Build history of the part. All positions in model axes, mm. Face numbers are marked on the shaded views. A direction names the side the tool comes from. Round coordinates to 2 decimals unless told otherwise and drop trailing zeros. Write each loop counter-clockwise with the first axis right and the second up, starting at its lowest first coordinate (ties: lowest second). Pieces come first, ordered by that corner, then holes.
Item 1: 3-axis set-ups, long thin cutter, end or side, ignore diameter. For the marked faces 4 and 5: which of +Z, -Z, +X, -X, +Y, -Y reach the whole face in a straight line?
Item 2: Drop flat-ended pins along their axis: pin 1 Ø6 at (y, z) = (23.5, 4.5) entering from -X; pin 2 Ø0.8 at (x, z) = (0.5, 10.5) entering from -Y; pin 3 Ø0.8 at (x, y) = (-25.5, -0.5) entering from -Z. Give the stop position or say it passes through.
Item 3: Band-saw the part on C-C, the plane z = 10. Write the cut outline in (x, y), then the cut area to 3 significant figures.
Item 4: Band-saw the part on D-D, the plane x = -23. Write the cut outline in (y, z).
Item 5: Band-saw the part on A-A, the plane x = -18. Write the cut outline in (y, z), then the cut area to 3 significant figures.
Item 6: Band-saw the part on B-B, the plane y = 15. Write the cut outline in (x, z), then the cut area to 3 significant figures.
Item 7: Wall check: probe 1 along X at (y, z) = (2.4, 10); probe 2 along Z at (x, y) = (-28.5, 5.5); probe 3 along Y at (x, z) = (-2.3, 10). Give the ranges that are in metal, low to high.
Item 8: Mould opens along X. For the marked faces 1, 2 and 3 say: +X half, -X half, draft (parallel to the pull), parting line (faces both ways), or undercut.
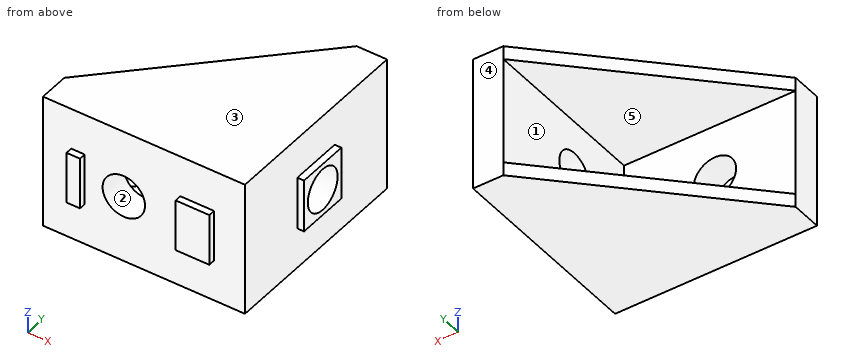
```python
from build123d import *

# Parameters (mm, degrees)
BOSS_EXTRUDE1_DEPTH = 20
CUT_EXTRUDE1_START  = -2
CUT_EXTRUDE1_DEPTH  = 16
SKETCH3_W           = 7.88
SKETCH3_H           = 7.88
BOSS_EXTRUDE2_DEPTH = 1
SKETCH4_R           = 3.15
CUT_EXTRUDE2_DEPTH  = 48.549973712
SKETCH5_W           = 2
SKETCH5_H           = 7.7
SKETCH5_W_2         = 5
BOSS_EXTRUDE3_DEPTH = 1
SKETCH6_R           = 3.15
CUT_EXTRUDE3_DEPTH  = 47.904157598


with BuildPart() as part:
    # Sketch1 → Boss-Extrude1 (new body)
    with BuildSketch(Plane.XY):
        Polygon((0, 0), (0, 30), (-4.5, 30), (-30, 4.5), (-30, 0), align=None)
    extrude(amount=BOSS_EXTRUDE1_DEPTH)

    # Sketch2 → Cut-Extrude1 (cut)
    with BuildSketch(Plane.XY.offset(20).offset(CUT_EXTRUDE1_START)):
        Polygon((-30, 4.5), (-4.5, 4.5), (-4.5, 30), align=None)
    extrude(amount=-CUT_EXTRUDE1_DEPTH, mode=Mode.SUBTRACT)

    # Sketch3 → Boss-Extrude2 (add)
    with BuildSketch(Plane(origin=(0, 0, 0), x_dir=(0, 0, -1), z_dir=(1, 0, 0))):
        with Locations((-10, 15)):
            Rectangle(SKETCH3_W, SKETCH3_H)
    extrude(amount=BOSS_EXTRUDE2_DEPTH)

    # Sketch4 → Cut-Extrude2 (cut, through all)
    with BuildSketch(Plane(origin=(1, 0, 0), x_dir=(0, 0, -1), z_dir=(1, 0, 0))):
        with Locations((-10, 15)):
            Circle(SKETCH4_R)
    extrude(amount=-CUT_EXTRUDE2_DEPTH, mode=Mode.SUBTRACT)

    # Sketch5 → Boss-Extrude3 (add)
    with BuildSketch(Plane.XZ):
        with Locations((-24.8, 10)):
            Rectangle(SKETCH5_W, SKETCH5_H)
        with Locations((-7.1, 10)):
            Rectangle(SKETCH5_W_2, SKETCH5_H)
    extrude(amount=BOSS_EXTRUDE3_DEPTH)

    # Sketch6 → Cut-Extrude3 (cut, through all)
    with BuildSketch(Plane.XZ):
        with Locations(Location((-18, 10, 0), (0, 0, 270))):
            Circle(SKETCH6_R)
    extrude(amount=-CUT_EXTRUDE3_DEPTH, mode=Mode.SUBTRACT)


solid = part.part
```
Results:
1. face 4: +Z, -Z, +X, -X, +Y
1. face 5: -X, +Y
2. pin 1: stops at x = -12.66
2. pin 2: stops at y = 11.06
2. pin 3: stops at z = 6.15
3. outline: (-30, 0) - (-25.8, 0) - (-25.8, -1) - (-23.8, -1) - (-23.8, 0) - (-21.15, 0) - (-21.15, 4.5) - (-30, 4.5) - close; (-14.85, 0) - (-9.6, 0) - (-9.6, -1) - (-4.6, -1) - (-4.6, 0) - (0, 0) - (0, 11.06) - (1, 11.06) - (1, 11.85) - (-4.5, 11.85) - (-4.5, 4.5) - (-14.85, 4.5) - close; (-4.5, 18.15) - (1, 18.15) - (1, 18.94) - (0, 18.94) - (0, 30) - (-4.5, 30) - close
3. area: 202 mm2
4. outline: (0, 0) - (11.5, 0) - (11.5, 2) - (4.5, 2) - (4.5, 18) - (11.5, 18) - (11.5, 20) - (0, 20) - close
5. outline: (0, 0) - (16.5, 0) - (16.5, 2) - (4.5, 2) - (4.5, 6.85) - (0, 6.85) - close; (0, 13.15) - (4.5, 13.15) - (4.5, 18) - (16.5, 18) - (16.5, 20) - (0, 20) - close
5. area: 110 mm2
6. outline: (-19.5, 0) - (0, 0) - (0, 6.06) - (1, 6.06) - (1, 6.85) - (-4.5, 6.85) - (-4.5, 2) - (-19.5, 2) - close; (-19.5, 18) - (-4.5, 18) - (-4.5, 13.15) - (1, 13.15) - (1, 13.94) - (0, 13.94) - (0, 20) - (-19.5, 20) - close
6. area: 123 mm2
7. probe 1: x = -30 to -21.15, -14.85 to 0
7. probe 2: z = 0 to 2, 18 to 20
7. probe 3: y = 0 to 11.85, 18.15 to 30
8. face 1: -X half
8. face 2: undercut
8. face 3: draft
